Study the drawing (mm; zero at the part's minimum x, y, z) and answer. Coordinates: 2 decimals unless noted, no trailing zeros. Loops run counter-clockwise (first coordinate to the right, second up) from the corner with the lowest first, then second, coordinate; pieces in that order, holes last.
Q1. Straight lines are drawn through the part: line 1 (Y direction, x = 3.5, z = 19.8); line 2 (Z direction, x = 5.5, y = 3.5); line 3 (X direction, y = 2, z = 8) (3 decimals). For each, find the intervals that lie inside material, in ascending order.
Q2. Flat-ended cylindrical pins translate along their axes: P1, Ø2, axis at x = 5.5, z = 11, coming from the +Y side; P2, Ø2.5, axis at x = 3, y = 4, coming from the -Z side; P3, Ø1.4, axis at x = 4.5, z = 6.5, coming from the -Y side. Find the tip coordinate at first contact, or state that the pin passes through.
Q3. Section D-D (x = 4.75) is taken. Give the vertices of the cut face in (y, z) (3 decimals).
Q4. Section C-C (z = 2) is taken. Give the vertices of the cut face in (x, y) (3 decimals), then the cut area to 3 significant figures.
Q5. The mould has two halves that part along X. Classify the marked faces 1, 2 and 3: pulls with the +X half, pulls with the -X half, needs draft (parallel to the pull), parting line crosses it, or undercut.
Q6. Section A-A (x = 3.5) is taken. Give the vertices of the cut face in (y, z) (3 decimals).
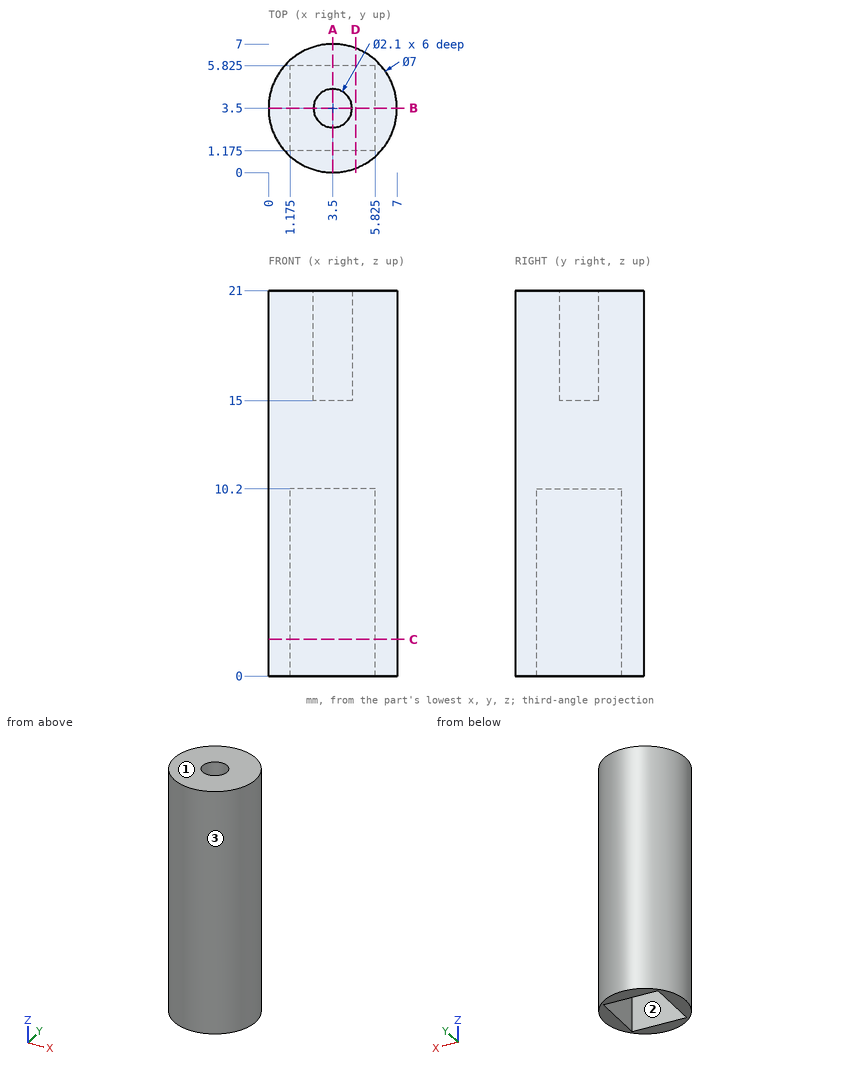
Numbers:
1. line 1: y = 0 to 2.45, 4.55 to 7
1. line 2: z = 10.2 to 21
1. line 3: x = 0.338 to 1.175, 5.825 to 6.662
2. P1: stops at y = 6.85
2. P2: stops at z = 10.2
2. P3: stops at y = 0.01
3. outline: (0.231, 0) - (1.175, 0) - (1.175, 10.2) - (5.825, 10.2) - (5.825, 0) - (6.769, 0) - (6.769, 21) - (0.231, 21) - close
4. outline: circle Ø7 at (3.5, 3.5); hole (1.175, 1.175) - (5.825, 1.175) - (5.825, 5.825) - (1.175, 5.825) - close
4. area: 16.9 mm2
5. face 1: needs draft
5. face 2: undercut
5. face 3: parting line crosses it
6. outline: (0, 0) - (1.175, 0) - (1.175, 10.2) - (5.825, 10.2) - (5.825, 0) - (7, 0) - (7, 21) - (4.55, 21) - (4.55, 15) - (2.45, 15) - (2.45, 21) - (0, 21) - close
